```python
from build123d import *

# Parameters (mm, degrees)
F1_DEPTH = 30
F2_DEPTH = 3.5
F3_DEPTH = 5
F4_SIZE  = 2
F5_R     = 3


# Not quite as in the source:
# - a feature names something its author has since deleted; it is built from what else it names


with BuildPart() as f1:
    # F0 (on Front) → F1 (new body)
    with BuildSketch(Plane.XZ):
        Polygon((5.4754310687, 0), (2.9508621374, 0), (1.3296836853, -11.5352840725), (3.8053538572, -11.8832168249), align=None)
        Polygon((10, 0), (7.4754310687, 0), (9.1455082802, -11.8832168249), (11.6211784521, -11.5352840725), align=None)
        Polygon((0, 3.5), (0, 0), (2.9508621374, 0), (5.4754310687, 0), (7.4754310687, 0), (10, 0), (12.5, 0), (15.5, 0), (20, 0), (20, 3.5), align=None)
    extrude(amount=F1_DEPTH)

    # F2 (cut): a face of the model
    f2_faces = [f1.faces().sort_by_distance(p)[0] for p in [
        (20, -15, 1.75),
    ]]
    extrude(f2_faces, amount=-F2_DEPTH, mode=Mode.SUBTRACT)

    # F3 (add): a face of the model
    f3_faces = [f1.faces().sort_by_distance(p)[0] for p in [
        (0, -15, 1.75),
    ]]
    extrude(f3_faces, amount=F3_DEPTH)

    # F4
    f4_edges = [f1.edges().sort_by_distance(p)[0] for p in [
        (11.621178, -15, -11.535284),
        (1.329684, -15, -11.535284),
    ]]
    chamfer(f4_edges, length=F4_SIZE)

    # F5
    f5_edges = [f1.edges().sort_by_distance(p)[0] for p in [
        (1.60803, -15, -9.554748),
        (11.342832, -15, -9.554748),
    ]]
    fillet(f5_edges, radius=F5_R)


solid = f1.part
```
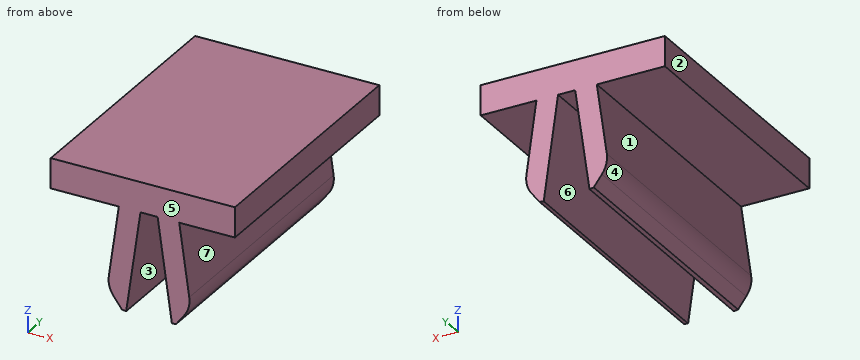
CAD build for the part. Positions are in the model's coordinates, mm. Face numbers are marked on the shaded views. A direction names the side the tool comes from. Round coordinates to 2 decimals unless told otherwise and drop trailing zeros. Write each loop counter-clockwise with the first axis right and the second up, starting at its lowest first coordinate (ties: lowest second). Pieces come first, ordered by that corner, then holes.
Item 1: Drop flat-ended pins along their axis: pin 1 Ø2.5 at (x, y) = (-0.5, -13) entering from -Z; pin 2 Ø1.5 at (y, z) = (-14.5, -9) entering from +X; pin 3 Ø8 at (x, z) = (13, -1.5) entering from -Y; pin 4 Ø3 at (y, z) = (-8, -4) entering from -X. Give the stop position or say it passes through.
Filled in:
pin 1: stops at z = 0
pin 2: stops at x = 11.2
pin 3: stops at y = -30
pin 4: stops at x = 2.18
Item 2: Band-saw the part on A-A on z = -4. Write the cut outline in (x, y).
Filled in:
outline: (2.39, -30) - (4.91, -30) - (4.91, 0) - (2.39, 0) - close; (8.04, -30) - (10.56, -30) - (10.56, 0) - (8.04, 0) - close
Item 3: Band-saw the part on C-C on x = 7. Write the cut outline in (y, z).
Filled in:
outline: (-30, 0) - (0, 0) - (0, 3.5) - (-30, 3.5) - close
Item 4: Drill centre lines: L1, parallel to Z at x = -2, y = -25.75; L2, parallel to X at y = -20.25, z = -4.25; L3, parallel to X at y = -13, z = -6.5. Where is each one in solid material? Low to high.
Filled in:
L1: z = 0 to 3.5
L2: x = 2.35 to 4.88, 8.07 to 10.6
L3: x = 2.04 to 4.56, 8.39 to 10.91
Item 5: Mould opens along Z. For the marked faces 1, 2, 3 and 4 say: released by +Z, released by -Z, zero draft, split by the parting line, or undercut.
Filled in:
face 1: undercut
face 2: zero draft
face 3: released by -Z
face 4: undercut
Item 6: Band-saw the part on B-B on y = -14.25. Write the cut outline in (x, z) (1 decimal), then the cut area to 3 significant figures.
Filled in:
outline: (-5, 0) - (3, 0) - (1.8, -8.3) arc R3 ccw to (2.4, -10.5) - (3.3, -11.8) - (3.8, -11.9) - (5.5, 0) - (7.5, 0) - (9.1, -11.9) - (9.6, -11.8) - (10.6, -10.5) arc R3 ccw to (11.2, -8.3) - (10, 0) - (16.5, 0) - (16.5, 3.5) - (-5, 3.5) - close
area: 130 mm2
Item 7: Tool access for the marked faces 5, 6 and 7: list every direction of +Z, -Z, +X, -X, +Y, -Y with a clear straight run to the whole face (end or side of a thin tool).
Filled in:
face 5: +Z, -Z, +X, -X, -Y
face 6: -Z, +Y, -Y
face 7: +X, +Y, -Y
